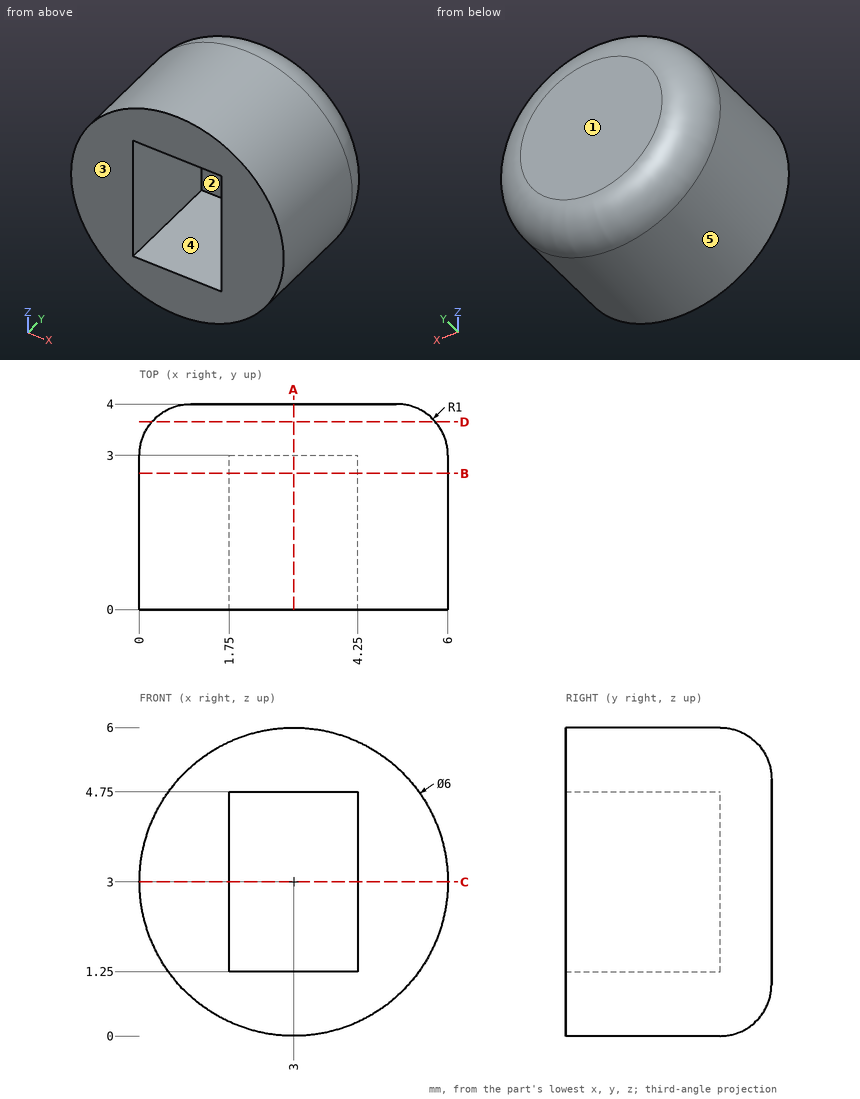
Drawing for the job (mm, zero at the part's lowest x, y, z). A direction names the side the tool comes from. Give positions to 0.01 mm unless a question says otherwise; leave off trailing zeros. Write each loop counter-clockwise with the first axis right and the second up, starting at its lowest first coordinate (ties: lowest second). Pieces come first, ordered by that corner, then holes. Notation, with made-up numbers: M 84.5,24 L 100.5,24 A18 cw 100.5,38 Z; hole C 51,27 d9. An arc over 180 degrees is marked long. Use CSV: the item, a comma, the result in double quotes.
Item 1: Drill centre lines: probe 1 along Y at (x, z) = (3.25, 1.9); probe 2 along X at (y, z) = (1.8, 4.35); probe 3 along Z at (x, y) = (2.5, 0.9). Where is each one in solid material? Low to high.
Taken from the geometry:
probe 1,"y = 3 to 4"
probe 2,"x = 0.32 to 1.75, 4.25 to 5.68"
probe 3,"z = 0.04 to 1.25, 4.75 to 5.96"
Item 2: Slice it at C-C on z = 3. Write the cut outline in (x, y).
Taken from the geometry:
outline,"M 0,0 L 1.75,0 L 1.75,3 L 4.25,3 L 4.25,0 L 6,0 L 6,3 A1 ccw 5,4 L 1,4 A1 ccw 0,3 Z"
Item 3: Pull direction X, two halves, no side cores. Call the marked faces 3, 4 and 5: +X half, -X half, draft (parallel to the pull), parting line (faces both ways), or undercut.
Taken from the geometry:
face 3,"draft"
face 4,"undercut"
face 5,"parting line"
Item 4: Slice it at A-A on x = 3. Write the cut outline in (y, z).
Taken from the geometry:
outline,"M 0,0 L 3,0 A1 ccw 4,1 L 4,5 A1 ccw 3,6 L 0,6 L 0,4.75 L 3,4.75 L 3,1.25 L 0,1.25 Z"
Item 5: Which spindle directions (+Z, -Z, +X, -X, +Y, -Y) get a long thin tool onto all of the face, cutting with end or side? Do the marked faces 1 and 2. Say none if no direction does.
Taken from the geometry:
face 1,"+Z, -Z, +X, -X, +Y"
face 2,"-Y"
Item 6: Slice it at D-D on y = 3.65. Write the cut outline in (x, z).
Taken from the geometry:
outline,"C 3,3 d5.52"
Item 7: Slice it at B-B on y = 2.65. Write the cut outline in (x, z).
Taken from the geometry:
outline,"C 3,3 d6; hole M 1.75,1.25 L 4.25,1.25 L 4.25,4.75 L 1.75,4.75 Z"
Item 8: Pin check, flat tip, straight feed: P1, Ø2, axis at x = 3, z = 3, coming from the -Y side. Stop position of the tip, or through.
Taken from the geometry:
P1,"stops at y = 3"
